from build123d import *

# Parameters (mm, degrees)
IZIM2_R               = 2.5
KES_EKSTR_ZYON1_DEPTH = 15.822873016
IZIM3_R               = 1
KES_EKSTR_ZYON3_DEPTH = 7
IZIM4_R               = 1.5
KES_EKSTR_ZYON4_DEPTH = 27
RADYUS1_R             = 0.2


with BuildPart() as part:
    # Çizim1 → Döndür1 (revolve)
    with BuildSketch(Plane.XY):
        with BuildLine():
            Line((0, 7), (0, 3.9))
            ThreePointArc((0, 3.9), (0.029289322, 3.829289322), (0.1, 3.8))
            Line((0.1, 3.8), (0.3, 3.8))
            Line((0.3, 3.8), (0, 3.5))
            Line((0, 3.5), (0, 0))
            Line((0, 0), (14.8, 0))
            Line((14.8, 0), (14.8, 1.887324991))
            Line((14.8, 1.887324991), (14.8, 3.6263585))
            Line((14.8, 3.6263585), (14.3, 4.1263585))
            Line((14.3, 4.1263585), (14, 4.1263585))
            Line((14, 4.1263585), (14, 6.1263585))
            Line((14, 6.1263585), (14.822873016, 7.772104531))
            Line((14.822873016, 7.772104531), (13.822873016, 7.772104531))
            Line((13.822873016, 7.772104531), (13, 6.1263585))
            Line((13, 6.1263585), (6, 6.1263585))
            Line((6, 6.1263585), (6, 7))
            Line((6, 7), (5.5, 8))
            Line((5.5, 8), (0.5, 8))
            Line((0.5, 8), (0, 7))
        make_face()
    revolve(axis=Axis((0, 0, 0), (1, 0, 0)))

    # Çizim2 → Kes-Ekstrüzyon1 (cut, through all)
    with BuildSketch(Plane.ZY):
        Circle(IZIM2_R)
    extrude(amount=-KES_EKSTR_ZYON1_DEPTH, mode=Mode.SUBTRACT)

    # Çizim3 → Kes-Ekstrüzyon3 (cut)
    with BuildSketch(Plane(origin=(6, 0, 0), x_dir=(0, 0, -1), z_dir=(1, 0, 0))):
        with Locations((6.1263585, 0)):
            Circle(IZIM3_R)
        with Locations((5.519658282, -2.658127333)):
            Circle(IZIM3_R)
        with Locations((3.819722047, -4.789779948)):
            Circle(IZIM3_R)
        with Locations((1.363243015, -5.972757901)):
            Circle(IZIM3_R)
        with Locations((-1.363243015, -5.972757901)):
            Circle(IZIM3_R)
        with Locations((-3.819722047, -4.789779948)):
            Circle(IZIM3_R)
        with Locations((-5.519658282, -2.658127333)):
            Circle(IZIM3_R)
        with Locations((-6.1263585, 0)):
            Circle(IZIM3_R)
        with Locations((-5.519658282, 2.658127333)):
            Circle(IZIM3_R)
        with Locations((-3.819722047, 4.789779948)):
            Circle(IZIM3_R)
        with Locations((-1.363243015, 5.972757901)):
            Circle(IZIM3_R)
        with Locations((1.363243015, 5.972757901)):
            Circle(IZIM3_R)
        with Locations((3.819722047, 4.789779948)):
            Circle(IZIM3_R)
        with Locations((5.519658282, 2.658127333)):
            Circle(IZIM3_R)
    extrude(amount=KES_EKSTR_ZYON3_DEPTH, mode=Mode.SUBTRACT)

    # Çizim4 → Kes-Ekstrüzyon4 (cut)
    with BuildSketch(Plane(origin=(0, 0, 0), x_dir=(1, 0, 0), z_dir=(0, 1, 0))):
        with Locations((3, 0)):
            Circle(IZIM4_R)
    extrude(amount=KES_EKSTR_ZYON4_DEPTH, mode=Mode.SUBTRACT)

    # Radyus1
    radyus1_edges = [part.edges().sort_by_distance(p)[0] for p in [
        (3, 7.858116823, 1.5),
        (1.5, 2.5, 0),
    ]]
    fillet(radyus1_edges, radius=RADYUS1_R)


solid = part.part
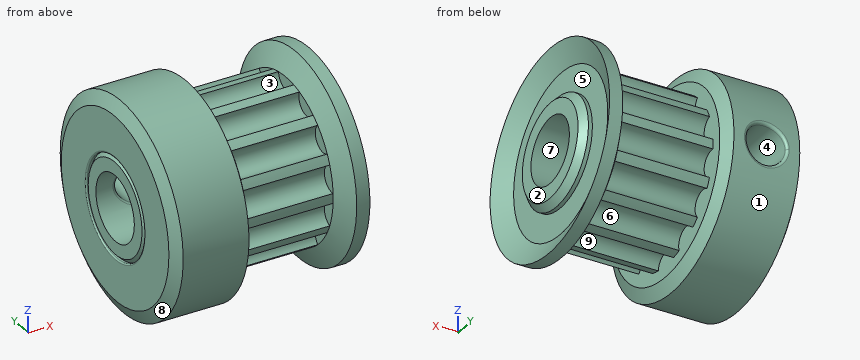
Build history of the part. All positions in model axes, mm. Face numbers are marked on the shaded views. A direction names the side the tool comes from. Give positions to 0.01 mm unless a question says otherwise; leave off trailing zeros. Write item = value, one per line. Start each with the question number.
1) Pull direction Y, two halves, no side cores. Call the marked faces 1, 2, 3 and 4: +Y half, -Y half, draft (parallel to the pull), parting line (faces both ways), or undercut.
2) Band-saw the part on B-B on y = 6.5. Count the separate pieces of the cut face and the enclosed holes in it, plus the area to 3 significant figures.
3) Tool access for the marked faces 5, 6, 7, 8 and 9: list every direction of +Z, -Z, +X, -X, +Y, -Y with a clear straight run to the whole face (end or side of a thin tool).
4) Probe probe 1 along X at (y, z) = (-5.75, 0.25); probe 2 along Y at (x, z) = (8.25, 0); probe 3 along Z at (x, y) = (8, -4.75). List the from-to ranges inside material, lowest first. Write a range as from..to.
5) Drop flat-ended pins along their axis: pin 1 Ø4 at (x, y) = (10, -6.5) entering from +Z; pin 2 Ø4 at (y, z) = (0, 0) entering from -X; pin 3 Ø6 at (y, z) = (0, 0) entering from +X; pin 4 Ø8 at (x, y) = (9, 3.5) entering from -Z. Give the stop position or say it passes through.
Final values:
q1.face_1 = parting line
q1.face_2 = undercut
q1.face_3 = undercut
q1.face_4 = draft
q2.separate_pieces = 2
q2.enclosed_holes = 1
q2.area = 55.5 mm²
q3.face_5 = +X
q3.face_6 = none
q3.face_7 = +X, -X
q3.face_8 = -X
q3.face_9 = -Z
q4.probe_1 = 0..14
q4.probe_2 = -6.13..-2.5, 2.5..6.13
q4.probe_3 = -2.82..2.82
q5.pin_1 = 2.99
q5.pin_2 = through
q5.pin_3 = 14.8
q5.pin_4 = -7.85
